Verification items for the finished model (mm, model axes). Face numbers are marked on the shaded views. A direction names the side the tool comes from. Round coordinates to 2 decimals unless told otherwise and drop trailing zeros. Loops run counter-clockwise (first coordinate to the right, second up) from the corner with the lowest first, then second, coordinate; pieces in that order, holes last. Notation, with made-up numbers: (-33.5, 5.5) - (-20.5, 5.5) arc R17 ccw to (-20.5, 36.5) - close; hole circle Ø3 at (51.5, 83.5). An arc over 180 degrees is marked (long way). Use CSV: the item, a comma, the result in double quotes.
Autodesk Inventor part; units mm, degrees
ref_plane "YZ Plane" through (0, 0, 0) normal (1, 0, 0) x (0, 1, 0)
ref_plane "XZ Plane" through (0, 0, 0) normal (0, 1, 0) x (-1, 0, 0)
ref_plane "XY Plane" through (0, 0, 0) normal (0, 0, 1) x (1, 0, 0)
sketch "Sketch1" plane through (0, 0, 0) normal (0, 0, 1) x (1, 0, 0)
  circle A0 centre (0, 0) radius 32
  circle A1 centre (0, 0) radius 2
  dimension "d0" = 64
  dimension "d1" = 4
extrude "Extrusion1" add sketch "Sketch1" along normal blind 20
sketch "Sketch2" plane through (0, 0, 20) normal (0, 0, 1) x (1, 0, 0)
  circle A0 centre (0, 0) radius 2
  circle A1 centre (0, 0) radius 10
  dimension "d4" = 20
extrude "Extrusion2" add sketch "Sketch2" along normal blind 7
sketch "Sketch3" plane through (0, 0, 20) normal (0, 0, 1) x (1, 0, 0)
  circle A0 centre (0, 0) radius 20
  dimension "d7" = 40
extrude "Extrusion3" add sketch "Sketch3" along normal blind 0.5
properties part number "weel" material "Rubber"
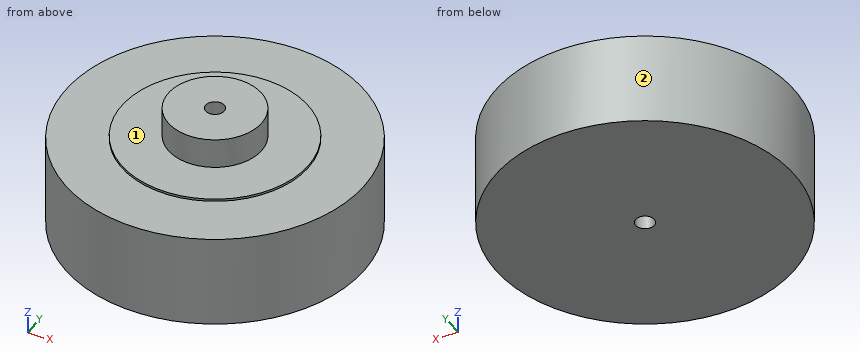
1) Gauge pin test, flat ends, axial feed: pin 1 Ø10 at (x, y) = (14, 8.5) entering from +Z; pin 2 Ø6 at (y, z) = (-5, 9.5) entering from -X; pin 3 Ø10 at (x, z) = (-5, 13.5) entering from +Y. Record the tip position at first contact, or that the pin passes through.
Returned:
pin 1,"stops at z = 20.5"
pin 2,"stops at x = -31.94"
pin 3,"stops at y = 32"
2) Thickness scan on probe 1 along X at (y, z) = (0, 25); probe 2 along Y at (x, z) = (0, 8); probe 3 along Z at (x, y) = (-20.5, -15). Record the ranges inside material, lowest first. Write a range as [from, to].
Returned:
probe 1,"x = [-10, -2], [2, 10]"
probe 2,"y = [-32, -2], [2, 32]"
probe 3,"z = [0, 20]"
3) Access from +Z, -Z, +X, -X, +Y, -Y to the whole of each face (thin tool, end or side, straight path). Record for the marked faces 1 and 2.
Returned:
face 1,"+Z"
face 2,"+Z, -Z"
4) Cross-section at D-D, the plane z = 23. Record the cut outline in (x, y).
Returned:
outline,"circle Ø20 at (0, 0); hole circle Ø4 at (0, 0)"
5) Cross-section at C-C, the plane z = 18. Record the cut outline in (x, y), then the cut area to 3 significant figures.
Returned:
outline,"circle Ø64 at (0, 0); hole circle Ø4 at (0, 0)"
area,"3,200 mm²"
6) Cross-section at A-A, the plane x = 0. Record the cut outline in (y, z).
Returned:
outline,"(-32, 0) - (-2, 0) - (-2, 20) - (2, 20) - (2, 0) - (32, 0) - (32, 20) - (20, 20) - (20, 20.5) - (10, 20.5) - (10, 27) - (2, 27) - (2, 20.5) - (-2, 20.5) - (-2, 27) - (-10, 27) - (-10, 20.5) - (-20, 20.5) - (-20, 20) - (-32, 20) - close"
